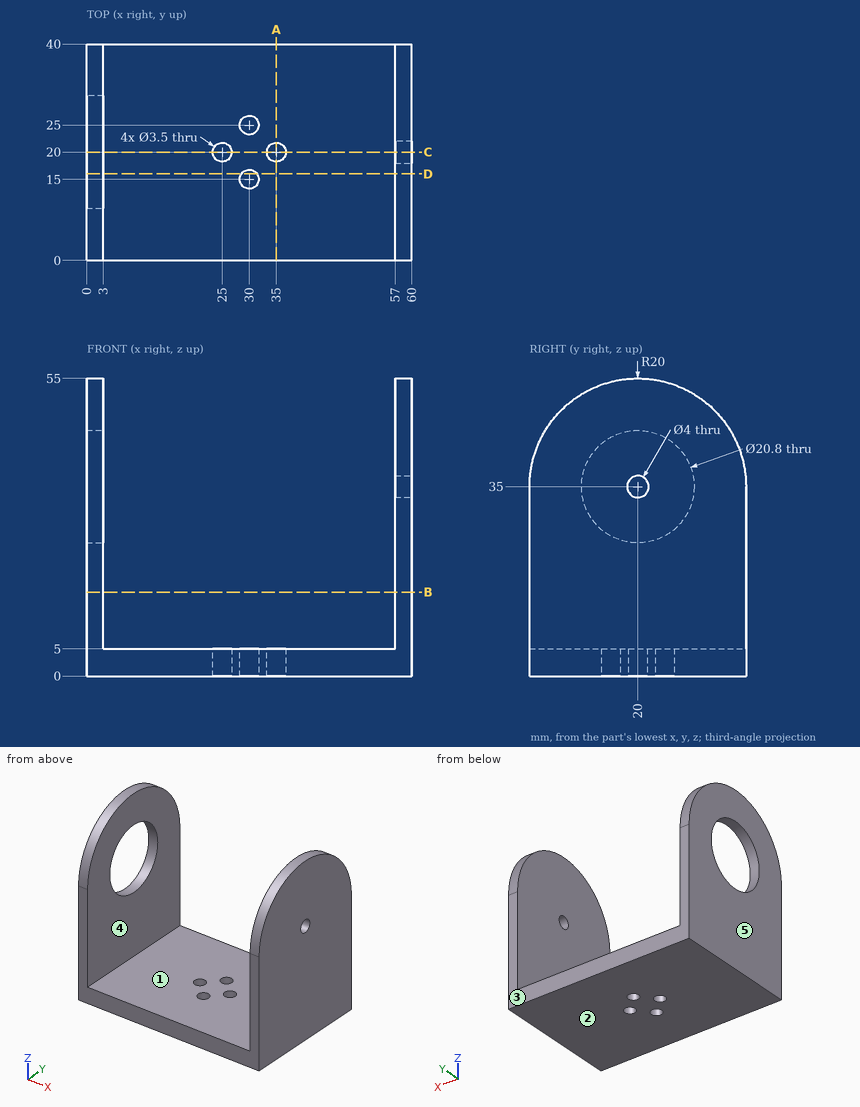
The drawing under review shows one solid part. Ordinate dimensions are in mm from its lowest x, y, z. A direction names the side the tool comes from. Coordinates: 2 decimals unless noted, no trailing zeros. Order: outer loops, then holes, each group sorted by start corner. A loop starts at its lowest first (then second) coordinate and runs counter-clockwise, first axis right, second up. Notation, with made-up numbers: (87, 71) -> (112, 71) arc R9 cw to (112, 80) -> close; hole circle Ø2 at (-6.75, 68.5). An arc over 180 degrees is marked (long way). Answer as CSV lines item,"result".
Q1. Draft analysis for pull direction X (two halves, no side actions). For the marked faces 3, 4 and 5, state which applies: released by +X, released by -X, zero draft, split by the parting line, or undercut.
Model answer:
face 3,"zero draft"
face 4,"undercut"
face 5,"released by -X"
Q2. We need section A-A (x = 35). State the section outline as (y, z) points.
Model answer:
outline,"(0, 0) -> (18.25, 0) -> (18.25, 5) -> (0, 5) -> close; (21.75, 0) -> (40, 0) -> (40, 5) -> (21.75, 5) -> close"
Q3. We need section C-C (y = 20). State the section outline as (x, z) points.
Model answer:
outline,"(0, 0) -> (23.25, 0) -> (23.25, 5) -> (3, 5) -> (3, 24.6) -> (0, 24.6) -> close; (0, 45.4) -> (3, 45.4) -> (3, 55) -> (0, 55) -> close; (26.75, 0) -> (33.25, 0) -> (33.25, 5) -> (26.75, 5) -> close; (36.75, 0) -> (60, 0) -> (60, 33) -> (57, 33) -> (57, 5) -> (36.75, 5) -> close; (57, 37) -> (60, 37) -> (60, 55) -> (57, 55) -> close"
Q4. For the marked faces 1 and 2, list the 3-axis set-ups (+Z, -Z, +X, -X, +Y, -Y) from which the entire face can be reached by the end or side of a thin tool; tool diameter is ignored.
Model answer:
face 1,"+Z, +Y, -Y"
face 2,"-Z, +X, -X, +Y, -Y"
Q5. We need section D-D (y = 16). State the section outline as (x, z) points.
Model answer:
outline,"(0, 0) -> (28.56, 0) -> (28.56, 5) -> (3, 5) -> (3, 25.4) -> (0, 25.4) -> close; (0, 44.6) -> (3, 44.6) -> (3, 54.6) -> (0, 54.6) -> close; (31.44, 0) -> (60, 0) -> (60, 54.6) -> (57, 54.6) -> (57, 5) -> (31.44, 5) -> close"
Q6. Clearance check with a flat-ended pin moving along its axis: pin 1 Ø5 at (x, y) = (49.5, 22) entering from +Z. State where the tip first meets the part, or that it passes through.
Model answer:
pin 1,"stops at z = 5"
Q7. We need section B-B (z = 15.5). State the section outline as (x, y) points, plus the area to 3 significant figures.
Model answer:
outline,"(0, 0) -> (3, 0) -> (3, 40) -> (0, 40) -> close; (57, 0) -> (60, 0) -> (60, 40) -> (57, 40) -> close"
area,"240 mm2"
Q8. Wall thickness on line 1 along Y through (x, z) = (30, 2.75); line 2 along X through (y, z) = (37.5, 21.5); line 3 along Z through (x, y) = (57.6, 20): over which ranges is each line inside the solid? List them lowest first. Write a range as [from, to].
Model answer:
line 1,"y = [0, 13.25], [16.75, 23.25], [26.75, 40]"
line 2,"x = [0, 3], [57, 60]"
line 3,"z = [0, 33], [37, 55]"
